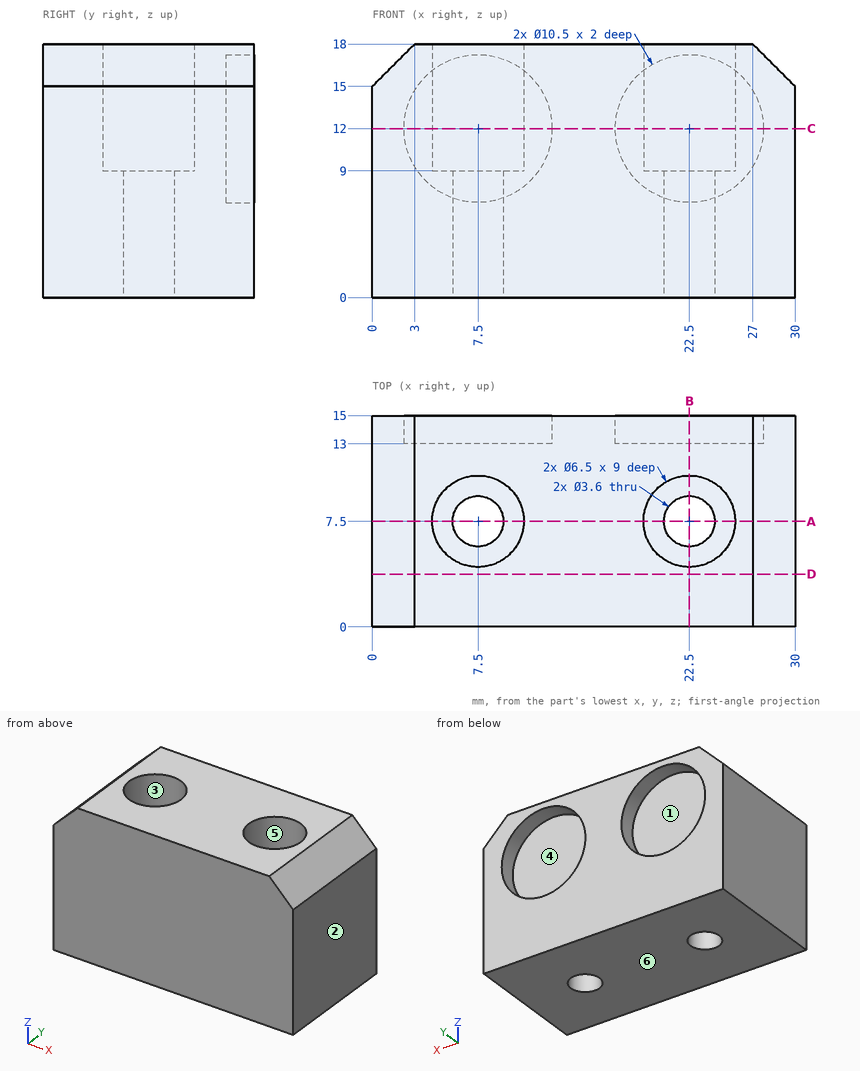
The drawing under review shows one solid part. Ordinate dimensions are in mm from its lowest x, y, z. A direction names the side the tool comes from. Give positions to 0.01 mm unless a question says otherwise; leave off trailing zeros. Order: outer loops, then holes, each group sorted by start corner. A loop starts at its lowest first (then second) coordinate and runs counter-clockwise, first axis right, second up. Notation, with made-up numbers: (59, -12) -> (74, -12) arc R12 ccw to (74, 11) -> close; hole circle Ø8 at (61, -37.75). An arc over 180 degrees is marked (long way). Write item = value, one per line.
1) Draft analysis for pull direction Y (two halves, no side actions). For the marked faces 4, 5 and 6, state which applies: pulls with the +Y half, pulls with the -Y half, needs draft (parallel to the pull), parting line crosses it, or undercut.
Findings:
face_4 = pulls with the +Y half
face_5 = undercut
face_6 = needs draft
2) For the marked faces 1, 2 and 3, list the 3-axis set-ups (+Z, -Z, +X, -X, +Y, -Y) from which the entire face can be reached by the end or side of a thin tool; tool diameter is ignored.
Findings:
face_1 = +Y
face_2 = +Z, -Z, +X, +Y, -Y
face_3 = +Z
3) We need section D-D, the plane y = 3.75. Give the boundary of the cut face in (x, z), and give its area (3 significant figures).
Findings:
outline = (0, 0) -> (30, 0) -> (30, 15) -> (27, 18) -> (3, 18) -> (0, 15) -> close
area = 531 mm^2
4) We need section B-B, the plane x = 22.5. Give the boundary of the cut face in (y, z).
Findings:
outline = (0, 0) -> (5.7, 0) -> (5.7, 9) -> (4.25, 9) -> (4.25, 18) -> (0, 18) -> close; (9.3, 0) -> (15, 0) -> (15, 6.75) -> (13, 6.75) -> (13, 17.25) -> (15, 17.25) -> (15, 18) -> (10.75, 18) -> (10.75, 9) -> (9.3, 9) -> close
5) We need section A-A, the plane y = 7.5. Give the boundary of the cut face in (x, z).
Findings:
outline = (0, 0) -> (5.7, 0) -> (5.7, 9) -> (4.25, 9) -> (4.25, 18) -> (3, 18) -> (0, 15) -> close; (9.3, 0) -> (20.7, 0) -> (20.7, 9) -> (19.25, 9) -> (19.25, 18) -> (10.75, 18) -> (10.75, 9) -> (9.3, 9) -> close; (24.3, 0) -> (30, 0) -> (30, 15) -> (27, 18) -> (25.75, 18) -> (25.75, 9) -> (24.3, 9) -> close
6) To check wall thickness, follow L1, parallel to X at y = 13.4, z = 12; L2, parallel to Y at x = 7.5, z = 4.5; L3, parallel to X at y = 6, z = 5.5. State the ranges of each line that lie inside material, in increasing order. Write a range as from..to.
Findings:
L1 = 0..2.25, 12.75..17.25, 27.75..30
L2 = 0..5.7, 9.3..15
L3 = 0..6.51, 8.49..21.51, 23.49..30
7) We need section C-C, the plane z = 12. Give the boundary of the cut face in (x, y).
Findings:
outline = (0, 0) -> (30, 0) -> (30, 15) -> (27.75, 15) -> (27.75, 13) -> (17.25, 13) -> (17.25, 15) -> (12.75, 15) -> (12.75, 13) -> (2.25, 13) -> (2.25, 15) -> (0, 15) -> close; hole circle Ø6.5 at (7.5, 7.5); hole circle Ø6.5 at (22.5, 7.5)
8) Insertion check: pin 1 (1.5 mm diameter, centred on x = 5, z = 11.5, fed in from +Y); pin 2 (3 mm diameter, centred on x = 7.5, y = 7.5, fed in from -Z); pin 3 (5 mm diameter, centred on x = 7.5, y = 7.5, fed in from +Z). Each pin has a flat end and moves straight along its axis. Give the tip position at first contact, or say it passes through.
Findings:
pin_1 = 13
pin_2 = through
pin_3 = 9
